Autodesk Inventor part; units mm, degrees
ref_plane "YZ Plane" through (0, 0, 0) normal (1, 0, 0) x (0, 1, 0)
ref_plane "XZ Plane" through (0, 0, 0) normal (0, 1, 0) x (-1, 0, 0)
ref_plane "XY Plane" through (0, 0, 0) normal (0, 0, 1) x (1, 0, 0)
sketch "Sketch1" plane through (0, 0, 0) normal (0, 1, 0) x (-1, 0, 0)
  line L0 (381, 15.875) -> (-381, 15.875)
  line L1 (-381, 15.875) -> (-381, -15.875)
  line L2 (-381, -15.875) -> (381, -15.875)
  line L3 (381, -15.875) -> (381, 15.875)
  point P0 (0, 0)
  dimension "d0" = 762
  dimension "d1" = 31.75
extrude "Extrusion1" add sketch "Sketch1" along normal blind 3.175
sketch "Sketch2" plane through (-381, 0, 15.875) normal (0, 0, 1) x (1, 0, 0)
  line L0 (0, 3.175) -> (762, 3.175)
  line L1 (762, 28.575) -> (0, 28.575)
  line L2 (0, 28.575) -> (0, 3.175)
  line L3 (0, 3.175) -> (762, 3.175)
  line L4 (762, 3.175) -> (762, 28.575)
  point P0 (381, 0)
extrude "Extrusion2" add sketch "Sketch2" against normal blind 3.175
sketch "Sketch3" plane through (-381, 28.575, 15.875) normal (0, 1, 0) x (1, 0, 0)
  line L0 (0, 3.175) -> (762, 3.175)
  line L1 (762, 28.575) -> (0, 28.575)
  line L2 (0, 28.575) -> (0, 3.175)
  line L3 (0, 3.175) -> (762, 3.175)
  line L4 (762, 3.175) -> (762, 28.575)
  point P0 (381, 15.875)
extrude "Extrusion3" add sketch "Sketch3" against normal blind 3.175
sketch "Sketch4" plane through (381, 28.575, -12.7) normal (0, 0, -1) x (-1, 0, 0)
  line L0 (762, 0) -> (0, 0)
  line L1 (0, -25.4) -> (762, -25.4)
  line L2 (0, -3.175) -> (0, -25.4)
  line L3 (762, -25.4) -> (762, -3.175)
  line L4 (762, 0) -> (0, 0)
  line L5 (0, 0) -> (0, -25.4)
  line L6 (0, -25.4) -> (762, -25.4)
  line L7 (762, -25.4) -> (762, 0)
  point P0 (381, -28.575)
extrude "Extrusion4" add sketch "Sketch4" along normal blind 3.175
sketch "Sketch5" plane through (-381, 28.575, 15.875) normal (0, 1, 0) x (1, 0, 0)
  line L0 (0, 31.75) -> (762, 31.75)
  line L1 (0, 0) -> (762, 0)
  line L2 (762, 0) -> (762, 31.75)
  line L3 (0, 31.75) -> (762, 31.75)
  line L4 (0, 0) -> (0, 31.75)
  line L5 (0, 31.75) -> (762, 31.75)
  line L6 (762, 31.75) -> (762, 0)
  line L7 (762, 0) -> (0, 0)
  line L8 (0, 0) -> (0, 31.75)
  point P0 (381, 15.875)
extrude "Extrusion5" add sketch "Sketch5" along normal blind 3.175
sketch "Sketch6" plane through (-381, 25.4, 15.875) normal (0, -1, 0) x (1, 0, 0)
  line L0 (0, -3.175) -> (0, -28.575)
  line L1 (0, -28.575) -> (762, -28.575)
  line L2 (762, -28.575) -> (762, -3.175)
  line L3 (0, -3.175) -> (762, -3.175)
  line L4 (762, -3.175) -> (0, -3.175)
  line L5 (0, -3.175) -> (0, -28.575)
  line L6 (0, -28.575) -> (762, -28.575)
  line L7 (762, -28.575) -> (762, -3.175)
  point P0 (381, -15.875)
extrude "Extrusion6" cut sketch "Sketch6" against normal blind 3.175
sketch "Sketch7" plane through (381, 0, 15.875) normal (1, 0, 0) x (0, 0, -1)
  line L0 (0, 31.75) -> (31.75, 31.75)
  line L1 (31.75, 0) -> (31.75, 31.75)
  line L2 (0, 31.75) -> (31.75, 31.75)
  line L3 (0, 0) -> (0, 31.75)
  line L4 (0, 0) -> (31.75, 0)
  line L5 (3.175, 28.575) -> (3.175, 3.175)
  line L6 (3.175, 28.575) -> (28.575, 28.575)
  line L7 (28.575, 28.575) -> (28.575, 3.175)
  line L8 (3.175, 3.175) -> (28.575, 3.175)
  line L9 (0, 0) -> (0, 31.75)
  line L10 (0, 31.75) -> (31.75, 31.75)
  line L11 (31.75, 31.75) -> (31.75, 0)
  line L12 (31.75, 0) -> (0, 0)
  line L13 (0, 0) -> (0, 31.75)
  line L14 (3.175, 28.575) -> (28.575, 28.575)
  line L15 (28.575, 28.575) -> (28.575, 3.175)
  line L16 (28.575, 3.175) -> (3.175, 3.175)
  line L17 (3.175, 3.175) -> (3.175, 28.575)
  point P0 (15.875, 0)
extrude "Extrusion7" cut sketch "Sketch7" against normal blind 254
properties part number "alignmentWheelsBarSolid"
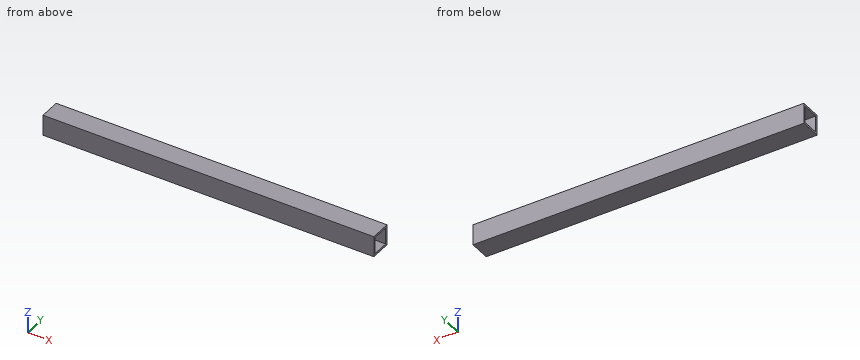
The model under review builds one solid part; all positions refer to its coordinate system, in mm. Round coordinates to 2 decimals unless told otherwise and drop trailing zeros. Loops run counter-clockwise (first coordinate to the right, second up) from the corner with the lowest first, then second, coordinate; pieces in that order, holes last. Notation, with made-up numbers: (-17.75, 35) -> (33.25, 35) arc R14 cw to (33.25, 57) -> close; hole circle Ø2 at (15, -31.75). An arc over 180 degrees is marked (long way). Answer as a JSON object with one key per item and string values. Group by question number.
1) We need section B-B on z = -0.5. Write out the cut boundary in (x, y) (3 decimals).
2) For line 1 (Z direction, x = -33, y = 28.5) (3 decimals); line 2 (Y direction, x = -26.5, z = 12) (3 decimals), list the stretches that pass through material, from the lowest coordinate up. Write a range as [from, to].
3) We need section A-A on x = -274. Write out the cut boundary in (y, z) (3 decimals).
4) We need section C-C on y = 23.5. Write out the cut boundary in (x, z) (3 decimals), then the cut area to 3 significant figures.
Result set:
{
 "1": {"outline": "(-381, 0) -> (127, 0) -> (127, 3.175) -> (-381, 3.175) -> close; (-381, 28.575) -> (127, 28.575) -> (127, 31.75) -> (-381, 31.75) -> close"},
 "2": {"line 1": "[-15.875, -12.7], [12.7, 15.875]", "line 2": "[0, 3.175], [28.575, 31.75]"},
 "3": {"outline": "(0, -15.875) -> (31.75, -15.875) -> (31.75, 15.875) -> (0, 15.875) -> close; hole (3.175, -12.7) -> (28.575, -12.7) -> (28.575, 12.7) -> (3.175, 12.7) -> close"},
 "4": {"outline": "(-381, -15.875) -> (127, -15.875) -> (127, -12.7) -> (-381, -12.7) -> close; (-381, 12.7) -> (127, 12.7) -> (127, 15.875) -> (-381, 15.875) -> close", "area": "3,230 mm²"}
}
